```python
from build123d import *

# Parameters (mm, degrees)
F0_R     = 46
F0_R_2   = 25
F1_DEPTH = 1.6
F2_R     = 1.5
F3_DEPTH = 25.4


with BuildPart() as f1:
    # F0 (on Top) → F1 (new body)
    with BuildSketch(Plane.XY):
        Circle(F0_R)
        Circle(F0_R_2, mode=Mode.SUBTRACT)
    extrude(amount=F1_DEPTH)

    # F2 (on face) → F3 (cut)
    with BuildSketch(Plane.XY.offset(1.6)):
        with Locations((0, 30)):
            Circle(F2_R)
        with Locations((-28.531695, 9.27051)):
            Circle(F2_R)
        with Locations((-17.633558, -24.27051)):
            Circle(F2_R)
        with Locations((17.633558, -24.27051)):
            Circle(F2_R)
        with Locations((28.531695, 9.27051)):
            Circle(F2_R)
    extrude(amount=-F3_DEPTH, mode=Mode.SUBTRACT)


solid = f1.part
```
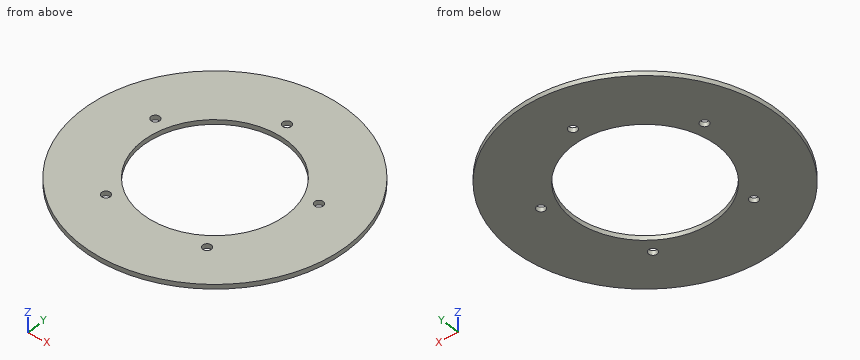
Here's how the part is built. I have some questions about the finished solid (model axes, mm). Coordinates: 2 decimals unless noted, no trailing zeros. Order: outer loops, then holes, each group sorted by start corner. A loop starts at its lowest first (then second) coordinate and runs counter-clockwise, first axis right, second up. Notation, with made-up numbers: M -26,64 L 19,64 A23 cw 19,85 Z; hole C -28.5,-35.75 d6. An arc over 180 degrees is marked long. Answer as a JSON object with one key per item and string values. Group by question number.
(1) Suppose I cut it at D-D, the plane x = -13.5. Please give me the cut outline in (y, z).
(2) Suppose I cut it at C-C, the plane z = 0.9. Please give me the cut outline in (x, y), then the cut area to 3 significant figures.
(3) For pin 1 (2.5 mm diameter, centred on x = 28.53, y = 9.27, fed in from -Z), with a flat end and sliding along its axis, tell me the tip position at first contact or that it passes through.
(4) Suppose I cut it at A-A, the plane y = 0. Please give me the cut outline in (x, z), then the cut area to 3 significant figures.
(5) Suppose I cut it at B-B, the plane x = 0. Please give me the cut outline in (y, z), then the cut area to 3 significant figures.
(6) I need wall thicknesses on probe 1 along Y at (x, z) = (0, 1.2); probe 2 along X at (y, z) = (8, 0.55); probe 3 along Y at (x, z) = (20.5, 0.4). Which ranges of each line are inside material? Lowest first, please.
Values found:
{
 "1": {"outline": "M -43.97,0 L -21.04,0 L -21.04,1.6 L -43.97,1.6 Z; M 21.04,0 L 43.97,0 L 43.97,1.6 L 21.04,1.6 Z"},
 "2": {"outline": "C 0,0 d92; hole C -28.53,9.27 d3; hole C 0,0 d50; hole C -17.63,-24.27 d3; hole C 0,30 d3; hole C 17.63,-24.27 d3; hole C 28.53,9.27 d3", "area": "4,650 mm^2"},
 "3": {"pin 1": "passes through"},
 "4": {"outline": "M -46,0 L -25,0 L -25,1.6 L -46,1.6 Z; M 25,0 L 46,0 L 46,1.6 L 25,1.6 Z", "area": "67.2 mm^2"},
 "5": {"outline": "M -46,0 L -25,0 L -25,1.6 L -46,1.6 Z; M 25,0 L 28.5,0 L 28.5,1.6 L 25,1.6 Z; M 31.5,0 L 46,0 L 46,1.6 L 31.5,1.6 Z", "area": "62.4 mm^2"},
 "6": {"probe 1": "y = -46 to -25, 25 to 28.5, 31.5 to 46", "probe 2": "x = -45.3 to -29.33, -27.73 to -23.69, 23.69 to 27.73, 29.33 to 45.3", "probe 3": "y = -41.18 to -14.31, 14.31 to 41.18"}
}
